Could you check a few things on this drawing? It's one solid part, dimensions in mm from its lowest x, y, z. Give positions to 0.01 mm unless a question says otherwise; leave off trailing zeros. Loops run counter-clockwise (first coordinate to the right, second up) from the corner with the lowest first, then second, coordinate; pieces in that order, holes last. Notation, with made-up numbers: M -11,3.5 L 13,3.5 A18 ccw 13,16.5 Z; hole C -8.5,40 d7. An arc over 180 degrees is marked long. Answer as a JSON object with one key per item and string values.
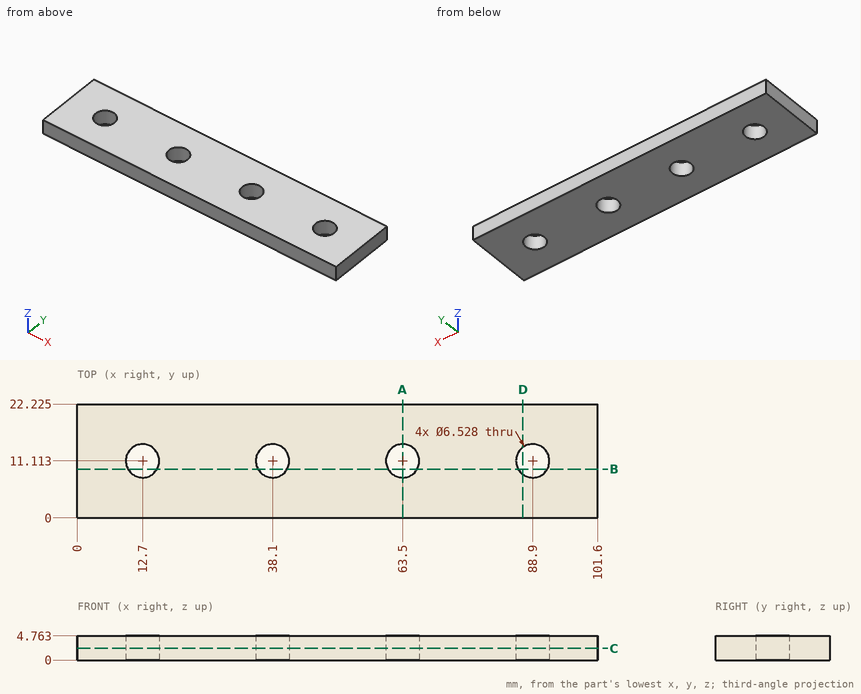
1) Please list where these lines run through material, in increasing order: line 1 along Y through (x, z) = (38.1, 3.05) (1 decimal); line 2 along X through (y, z) = (9.5, 2.45); line 3 along X through (y, z) = (13.5, 1.9) (1 decimal). Write a range as from..to.
Answer list:
{"line 1": "0..7.8, 14.4..22.2", "line 2": "0..9.86, 15.54..35.26, 40.94..60.66, 66.34..86.06, 91.74..101.6", "line 3": "0..10.5, 14.9..35.9, 40.3..61.3, 65.7..86.7, 91.1..101.6"}
2) Suppose I cut it at B-B, the plane y = 9.5. Write out the boundary of the cut face in (x, z).
Answer list:
{"outline": "M 0,0 L 9.86,0 L 9.86,4.76 L 0,4.76 Z; M 15.54,0 L 35.26,0 L 35.26,4.76 L 15.54,4.76 Z; M 40.94,0 L 60.66,0 L 60.66,4.76 L 40.94,4.76 Z; M 66.34,0 L 86.06,0 L 86.06,4.76 L 66.34,4.76 Z; M 91.74,0 L 101.6,0 L 101.6,4.76 L 91.74,4.76 Z"}
3) Suppose I cut it at D-D, the plane x = 87. Write out the boundary of the cut face in (y, z) (1 decimal).
Answer list:
{"outline": "M 0,0 L 8.5,0 L 8.5,4.8 L 0,4.8 Z; M 13.8,0 L 22.2,0 L 22.2,4.8 L 13.8,4.8 Z"}
4) Suppose I cut it at A-A, the plane x = 63.5. Write out the boundary of the cut face in (y, z) (1 decimal).
Answer list:
{"outline": "M 0,0 L 7.8,0 L 7.8,4.8 L 0,4.8 Z; M 14.4,0 L 22.2,0 L 22.2,4.8 L 14.4,4.8 Z"}
5) Suppose I cut it at C-C, the plane z = 2.3. Write out the boundary of the cut face in (x, y) (1 decimal).
Answer list:
{"outline": "M 0,0 L 101.6,0 L 101.6,22.2 L 0,22.2 Z; hole C 12.7,11.1 d6.5; hole C 38.1,11.1 d6.5; hole C 63.5,11.1 d6.5; hole C 88.9,11.1 d6.5"}
6) Will these pins go through, and if not, where does the flat tip stop? pin 1 Ø10 at (x, y) = (25, 10) entering from -Z; pin 2 Ø5 at (x, y) = (63.5, 11.11) entering from +Z.
Answer list:
{"pin 1": "z = 0", "pin 2": "through"}
